For this review, take the finished solid that the model builds, in its own axes (mm). Coordinates: 2 decimals unless noted, no trailing zeros. Loops run counter-clockwise (first coordinate to the right, second up) from the corner with the lowest first, then second, coordinate; pieces in that order, holes last. Notation, with made-up numbers: M -22.75,-31 L -2.75,-31 A12 ccw -2.75,-14 Z; hole C -15.75,0.5 d7. An arc over 180 degrees is marked long. Answer as a JSON object with one key per item and string values. Group by question number.
Item 1: Add section B-B (y = 101). State the section outline as (x, z) points (3 decimals), then the cut area to 3 significant figures.
Item 2: Add section D-D (x = 287.02). State the section outline as (y, z) points (3 decimals), then the cut area to 3 significant figures.
Item 3: Add section A-A (x = 230.5). State the section outline as (y, z) points (3 decimals).
Item 4: Wall thickness on L1, parallel to Y at x = 27.94, z = 1.5; L2, parallel to Y at x = 287.02, z = 2; L3, parallel to Y at x = 230.5, z = 1.9: over which ranges is each line inside the solid? List them lowest first. Write a range as from..to.
Item 5: Add section C-C (y = 17.78). State the section outline as (x, z) points (3 decimals), then the cut area to 3 significant figures.
Item 6: Insertion check: pin 1 (1.6 mm diameter, centred on x = 279.5, z = 1.5, fed in from -Y). The pin has a flat end and moves straight along its axis. Give the tip position at first contact, or say it passes through.
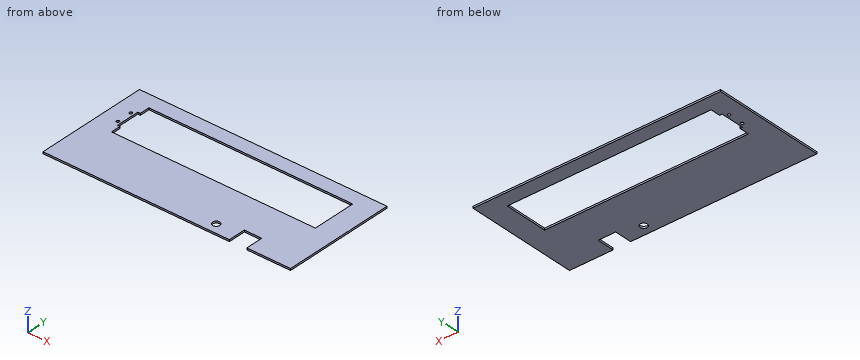
Autodesk Inventor part; units mm, degrees
ref_plane "YZ Plane" through (0, 0, 0) normal (1, 0, 0) x (0, 1, 0)
ref_plane "XZ Plane" through (0, 0, 0) normal (0, 1, 0) x (-1, 0, 0)
ref_plane "XY Plane" through (0, 0, 0) normal (0, 0, 1) x (1, 0, 0)
sketch "Sketch1" plane through (0, 0, 0) normal (0, 0, 1) x (1, 0, 0)
  line L0 (0, 0) -> (431.8, 0)
  line L1 (431.8, 0) -> (431.8, 196.85)
  line L2 (431.8, 196.85) -> (0, 196.85)
  line L3 (0, 196.85) -> (0, 0)
  line L4 (431.8, 0) -> (330.2, 0)
  line L5 (330.2, 0) -> (287.02, 0)
  line L6 (325.12, 0) -> (325.12, 30.48)
  line L7 (325.12, 30.48) -> (355.6, 30.48)
  line L8 (355.6, 30.48) -> (355.6, 0)
  line L9 (38.1, 171.45) -> (393.7, 171.45)
  line L10 (393.7, 171.45) -> (393.7, 95.25)
  line L11 (393.7, 95.25) -> (38.1, 95.25)
  line L12 (38.1, 95.25) -> (38.1, 171.45)
  line L13 (0, 196.85) -> (25.4, 196.85)
  line L14 (431.8, 196.85) -> (406.4, 196.85)
  line L15 (0, 196.85) -> (38.1, 196.85)
  line L16 (38.1, 196.85) -> (38.1, 171.45)
  line L17 (431.8, 0) -> (355.6, 0)
  line L18 (355.6, 0) -> (330.2, 0)
  line L19 (325.12, 0) -> (287.02, 0)
  point P0 (325.12, 0)
  dimension "d0" = 431.8
  dimension "d5" = 30.48
  dimension "d6" = 30.48
  dimension "d7" = 355.6
  dimension "d8" = 76.2
  dimension "d9" = 25.4
  dimension "d15" = 38.1
  dimension "d16" = 76.2
  dimension "d18" = 38.1
extrude "Extrusion1" add sketch "Sketch1" along normal blind 3.175 contours L3 L2 L1 L0 L8 L7 L6
sketch "Sketch2" plane through (0, 0, 3.175) normal (0, 0, 1) x (1, 0, 0)
  line L0 (0, 0) -> (325.12, 0)
  circle A0 centre (27.94, 120.142) radius 2.54
  circle A1 centre (27.94, 146.558) radius 2.54
  line L1 (38.1, 171.45) -> (393.7, 171.45)
  line L2 (38.1, 171.45) -> (38.1, 152.4)
  line L3 (38.1, 95.25) -> (38.1, 171.45)
  line L4 (38.1, 95.25) -> (38.1, 171.45)
  line L5 (38.1, 171.45) -> (38.1, 133.35)
  line L6 (287.02, 0) -> (287.02, 17.78)
  circle A2 centre (287.02, 17.78) radius 6.35
  dimension "d44" = 17.78
  dimension "d45" = 12.7
extrude "Extrusion2" cut sketch "Sketch2" against normal blind 25.4
sketch "Sketch4" plane through (0, 0, 3.175) normal (0, 0, 1) x (1, 0, 0)
  circle A0 centre (27.94, 146.558) radius 2.54
  line L0 (27.94, 146.558) -> (27.94, 152.4)
  line L1 (27.94, 152.4) -> (38.1, 152.4)
  line L2 (38.1, 95.25) -> (38.1, 171.45)
  line L3 (38.1, 152.4) -> (38.1, 114.3)
  line L4 (38.1, 114.3) -> (27.94, 114.3)
  circle A1 centre (27.94, 120.142) radius 2.54
  line L5 (27.94, 114.3) -> (27.94, 120.142)
  line L6 (38.1, 152.4) -> (35.56, 152.4)
  line L7 (35.56, 152.4) -> (35.56, 114.3)
  point P0 (0, 0)
  dimension "d30" = 5.842
  dimension "d31" = 38.1
  dimension "d32" = 2.54
extrude "Extrusion3" cut sketch "Sketch4" against normal blind 25.4 contours L1 L2 L4 L7
sketch "Sketch6" plane through (0, 0, 3.175) normal (0, 0, 1) x (1, 0, 0)
  line L0 (38.1, 152.4) -> (38.1, 171.45)
  line L1 (35.56, 153.9875) -> (38.1, 153.9875)
  line L2 (38.1, 153.9875) -> (38.1, 112.7125)
  line L3 (38.1, 112.7125) -> (33.7312, 112.7125)
  line L4 (33.7312, 112.7125) -> (33.7312, 153.9875)
  line L5 (33.7312, 153.9875) -> (35.56, 153.9875)
  point P0 (0, 0)
  dimension "d40" = 41.275
  dimension "d41" = 4.3688
extrude "Extrusion4" cut sketch "Sketch6" against normal blind 25.4
properties part number "220228 Back Piece"
From the geometry:
{
 "1": {"outline": "M 0,0 L 38.1,0 L 38.1,3.175 L 0,3.175 Z; M 393.7,0 L 431.8,0 L 431.8,3.175 L 393.7,3.175 Z", "area": "242 mm²"},
 "2": {"outline": "M 0,0 L 11.43,0 L 11.43,3.175 L 0,3.175 Z; M 24.13,0 L 95.25,0 L 95.25,3.175 L 24.13,3.175 Z; M 171.45,0 L 196.85,0 L 196.85,3.175 L 171.45,3.175 Z", "area": "343 mm²"},
 "3": {"outline": "M 0,0 L 95.25,0 L 95.25,3.175 L 0,3.175 Z; M 171.45,0 L 196.85,0 L 196.85,3.175 L 171.45,3.175 Z"},
 "4": {"L1": "y = 0..117.6, 122.68..144.02, 149.1..196.85", "L2": "y = 0..11.43, 24.13..95.25, 171.45..196.85", "L3": "y = 0..95.25, 171.45..196.85"},
 "5": {"outline": "M 0,0 L 280.67,0 L 280.67,3.175 L 0,3.175 Z; M 293.37,0 L 325.12,0 L 325.12,3.175 L 293.37,3.175 Z; M 355.6,0 L 431.8,0 L 431.8,3.175 L 355.6,3.175 Z", "area": "1,230 mm²"},
 "6": {"pin 1": "stops at y = 0"}
}
